from build123d import *

# Parameters (mm, degrees)
F1_R      = 30
F2_DEPTH  = 60
F4_DEPTH  = 60
F6_DEPTH  = 15
F8_DEPTH  = 60
F10_DEPTH = 30.001
F14_DEPTH = 30.001


with BuildPart() as f2:
    # F1 (on Front) → F2 (new body)
    with BuildSketch(Plane.XZ):
        Circle(F1_R)
    extrude(amount=F2_DEPTH)

    # F3 (on face) → F4 (cut, through all)
    with BuildSketch(Plane.XZ.offset(60)):
        with BuildLine():
            Line((30, 0), (-30, 0))
            ThreePointArc((-30, 0), (0, -30.0890051065), (30, 0))
        make_face()
    extrude(amount=-F4_DEPTH, mode=Mode.SUBTRACT)

    # F5 (on Top) → F6 (join)
    with BuildSketch(Plane.XY):
        with BuildLine():
            ThreePointArc((-38.9062538743, 0), (-48.9062538743, -10), (-38.9062538743, -20))
            Line((-38.9062538743, -20), (38.9062538743, -20))
            ThreePointArc((38.9062538743, -20), (48.9062538743, -10), (38.9062538743, 0))
            Line((38.9062538743, 0), (-38.9062538743, 0))
        make_face()
    extrude(amount=F6_DEPTH)

    # F7 (on face) → F8 (cut, through all)
    with BuildSketch(Plane.XZ.offset(60)):
        with BuildLine():
            Line((-25, 0), (25, 0))
            ThreePointArc((25, 0), (0, 25), (-25, 0))
        make_face()
    extrude(amount=-F8_DEPTH, mode=Mode.SUBTRACT)

    # F9 (on Top) → F10 (cut, through all)
    with BuildSketch(Plane.XY):
        with BuildLine():
            ThreePointArc((-35, -10), (-36.4644660941, -6.4644660941), (-40, -5))
            ThreePointArc((-40, -5), (-43.5355339059, -13.5355339059), (-35, -10))
        make_face()
        with BuildLine():
            ThreePointArc((45, -10), (43.5355339059, -6.4644660941), (40, -5))
            ThreePointArc((40, -5), (36.4644660941, -13.5355339059), (45, -10))
        make_face()
    extrude(amount=F10_DEPTH, mode=Mode.SUBTRACT)

    # F13 (on plane+point) → F14 (cut, through all)
    with BuildSketch(Plane.XY.offset(30)):
        with BuildLine():
            ThreePointArc((10, -40), (7.0710678119, -32.9289321881), (0, -30))
            Line((0, -30), (0, -60))
            Line((0, -60), (10, -60))
            Line((10, -60), (10, -40))
        make_face()
        with BuildLine():
            Line((0, -60), (0, -30))
            ThreePointArc((0, -30), (-7.0710678119, -32.9289321881), (-10, -40))
            Line((-10, -40), (-10, -60))
            Line((-10, -60), (0, -60))
        make_face()
    extrude(amount=-F14_DEPTH, mode=Mode.SUBTRACT)


solid = f2.part
Work out the finished part from the listing and answer in its coordinate system (mm). A direction names the side the tool comes from. Give positions to 0.01 mm unless a question says otherwise; leave off trailing zeros. Order: outer loops, then holes, each group sorted by start corner. A loop starts at its lowest first (then second) coordinate and runs counter-clockwise, first axis right, second up. Notation, with made-up numbers: (32.5, 79.5) - (73.5, 79.5) arc R20 ccw to (73.5, 116.5) - close; hole circle Ø2 at (50, 35). An arc over 180 degrees is marked (long way). Answer as CSV lines item,"result". Start each with the question number.
Q1. The mould has two halves that part along X. Classify faces 1 (the face through (3, 0, 25)), 2 (the face through (-48.904, -9.78, 7.395)), 3 (the face through (48.904, -10.22, 7.395)), 4 (the face through (0.55, -23.753, 24.994)): +X half, -X half, draft (parallel to the pull), parting line (faces both ways), or undercut.
Q2. Given pin 1 Ø6 at (x, y) = (32.5, -10) entering from +Z; pin 2 Ø8 at (x, y) = (22.5, -53) entering from +Z; pin 3 Ø2.5 at (y, z) = (-51.5, 26) entering from -X; pin 4 Ø13 at (x, y) = (40, -10) entering from -Z, each flat-ended and moving along its own axis, determine where each tip first touches the part or whether it passes through.
Q3. For faces 5 (the face through (34.7, -9.9, 15)), 6 (the face through (0.66, -29.58, 29.993)), 7 (the face through (10, -50, 26)), 8 (the face through (34, -20, 7)), determine the directions among +Z, -Z, +X, -X, +Y, -Y from which every point of the face is accessible in a straight line to the end or side of a thin tool.
Q4. The part is cut by section B-B (y = -52.5). Write down the section's boundary in (x, z), then the cut area to 3 significant figures.
Q5. The part is cut by section A-A (z = 9). Write down the section's boundary in (x, y), then the cut area to 3 significant figures.
Q6. The part is cut by section C-C (z = 24). Write down the section's boundary in (x, y), then the cut area to 3 significant figures.
Q7. The part is cut by section D-D (y = -9). Write down the section's boundary in (x, z).
Q8. Find the intervals of material crossed by L1, parallel to X at y = -10, z = 12.25; L2, parallel to X at y = -10, z = 3.75; L3, parallel to Y at x = 32.5, z = 6.5, in increasing order. Write a range as [from, to].
Check result:
1,face 1,"draft"
1,face 2,"-X half"
1,face 3,"+X half"
1,face 4,"undercut"
2,pin 1,"stops at z = 15"
2,pin 2,"stops at z = 23.62"
2,pin 3,"stops at x = -16.95"
2,pin 4,"stops at z = 0"
3,face 5,"+Z, +X, +Y, -Y"
3,face 6,"+Z, -Y"
3,face 7,"+Z, -Z, -Y"
3,face 8,"+Z, +X, -Y"
4,outline,"(-30, 0) - (-25, 0) arc R25 cw to (-10, 22.91) - (-10, 28.28) arc R30 ccw to start; (10, 22.91) arc R25 cw to (25, 0) - (30, 0) arc R30 ccw to (10, 28.28) - close"
4,area,"330 mm²"
5,outline,"(-38.91, -20) - (-28.62, -20) - (-28.62, -60) - (-23.32, -60) - (-23.32, 0) - (-38.91, 0) arc R10 ccw to start; (23.32, -60) - (28.62, -60) - (28.62, -20) - (38.91, -20) arc R10 ccw to (38.91, 0) - (23.32, 0) - close; hole circle Ø10 at (-40, -10); hole circle Ø10 at (40, -10)"
5,area,"1,200 mm²"
6,outline,"(-18, -60) - (-10, -60) - (-10, -40) arc R10 cw to (-7, -32.86) - (-7, 0) - (-18, 0) - close; (7, -32.86) arc R10 cw to (10, -40) - (10, -60) - (18, -60) - (18, 0) - (7, 0) - close"
6,area,"1,170 mm²"
7,outline,"(-48.86, 0) - (-44.9, 0) - (-44.9, 15) - (-48.86, 15) - close; (-35.1, 0) - (-25, 0) arc R25 cw to (25, 0) - (35.1, 0) - (35.1, 15) - (25.98, 15) arc R30 ccw to (-25.98, 15) - (-35.1, 15) - close; (44.9, 0) - (48.86, 0) - (48.86, 15) - (44.9, 15) - close"
8,L1,"x = [-48.91, -45], [-35, -21.79], [21.79, 35], [45, 48.91]"
8,L2,"x = [-48.91, -45], [-35, -24.72], [24.72, 35], [45, 48.91]"
8,L3,"y = [-20, 0]"
